For this review, take the finished solid that the model builds, in its own axes (mm). Round coordinates to 2 decimals unless told otherwise and drop trailing zeros. Write each loop counter-clockwise with the first axis right and the second up, starting at its lowest first coordinate (ties: lowest second). Pieces come first, ordered by that corner, then holes. Notation, with made-up numbers: M 61,84.25 L 104,84.25 A13 cw 104,103.25 Z; hole C 13,74.25 d2. An arc over 180 degrees is marked long. Use one line per item in the form item = value. Start each with the question number.
Item 1: For line 1 (X direction, y = 34.5, z = 1.8); line 2 (Y direction, x = 7, z = 2.25); line 3 (X direction, y = 5, z = 1.8), list the stretches that pass through material, from the lowest coordinate up. Write a range as [from, to].
Item 2: Draft analysis for pull direction Z (two halves, no side actions). For faces 1 (the flat face through (35, 22, 3)), 2 (the flat face through (69, 22, 2)), 3 (the flat face through (35, 22, 0)), state which applies: released by +Z, released by -Z, zero draft, split by the parting line, or undercut.
Item 3: For P1, Ø1.5, axis at x = 8.5, z = 2, coming from the +Y side, flat-tipped, find the tip position at first contact; note if it passes through.
Item 4: Add section A-A (z = 2.2). State the section outline as (x, y) points.
Autodesk Inventor part; units mm, degrees
ref_plane "YZ Plane" through (0, 0, 0) normal (1, 0, 0) x (0, 1, 0)
ref_plane "XZ Plane" through (0, 0, 0) normal (0, 1, 0) x (-1, 0, 0)
ref_plane "XY Plane" through (0, 0, 0) normal (0, 0, 1) x (1, 0, 0)
sketch "Boceto1" plane through (0, 0, 0) normal (0, 0, 1) x (1, 0, 0)
  line L0 (3, 0) -> (67, 0)
  line L1 (70, 3) -> (70, 41)
  line L2 (67, 44) -> (3, 44)
  line L3 (0, 41) -> (0, 3)
  arc A0 (3, 44) -> (0, 41) centre (3, 41) ccw
  arc A1 (0, 3) -> (3, 0) centre (3, 3) ccw
  arc A2 (67, 0) -> (70, 3) centre (67, 3) ccw
  arc A3 (70, 41) -> (67, 44) centre (67, 41) ccw
  point P0 (0, 0)
  point P1 (70, 44)
  point P2 (70, 0)
  point P3 (0, 44)
  dimension "d0" = 70
  dimension "d1" = 44
  dimension "d2" = 3
extrude "Extrusión1" add sketch "Boceto1" along normal blind 3
sketch "Boceto2" plane through (0, 0, 3) normal (0, 0, 1) x (1, 0, 0)
  line L0 (0, 41) -> (0, 3)
  arc A0 (0, 3) -> (3, 0) centre (3, 3) ccw
  line L1 (3, 0) -> (67, 0)
  arc A1 (67, 0) -> (70, 3) centre (67, 3) ccw
  line L2 (70, 3) -> (70, 41)
  arc A2 (70, 41) -> (67, 44) centre (67, 41) ccw
  line L3 (67, 44) -> (3, 44)
  arc A3 (3, 44) -> (0, 41) centre (3, 41) ccw
  line L4 (3, 43) -> (67, 43)
  arc A4 (69, 41) -> (67, 43) centre (67, 41) ccw
  line L5 (69, 41) -> (69, 3)
  arc A5 (67, 1) -> (69, 3) centre (67, 3) ccw
  line L6 (67, 1) -> (3, 1)
  arc A6 (1, 3) -> (3, 1) centre (3, 3) ccw
  line L7 (1, 3) -> (1, 41)
  arc A7 (3, 43) -> (1, 41) centre (3, 41) ccw
  point P0 (0, 0)
  dimension "d5" = 1
extrude "Extrusión2" cut sketch "Boceto2" against normal through all
sketch "Boceto5" plane through (0, 0, 3) normal (0, 0, 1) x (1, 0, 0)
  arc A0 (3, 43) -> (1, 41) centre (3, 41) ccw
  line L0 (1, 41) -> (1, 3)
  arc A1 (1, 3) -> (3, 1) centre (3, 3) ccw
  line L1 (3, 1) -> (67, 1)
  arc A2 (67, 1) -> (69, 3) centre (67, 3) ccw
  line L2 (69, 3) -> (69, 41)
  arc A3 (69, 41) -> (67, 43) centre (67, 41) ccw
  line L3 (67, 43) -> (3, 43)
  arc A4 (2.1716, 37.0858) -> (1, 34.2574) centre (5, 34.2574) ccw
  line L4 (1, 34.2574) -> (1, 9.7426)
  arc A5 (1, 9.7426) -> (2.1716, 6.9142) centre (5, 9.7426) ccw
  line L5 (2.1716, 6.9142) -> (6.9142, 2.1716)
  arc A6 (6.9142, 2.1716) -> (9.7426, 1) centre (9.7426, 5) ccw
  line L6 (9.7426, 1) -> (60.2574, 1)
  arc A7 (60.2574, 1) -> (63.0858, 2.1716) centre (60.2574, 5) ccw
  line L7 (63.0858, 2.1716) -> (67.8284, 6.9142)
  arc A8 (67.8284, 6.9142) -> (69, 9.7426) centre (65, 9.7426) ccw
  line L8 (69, 9.7426) -> (69, 34.2574)
  arc A9 (69, 34.2574) -> (67.8284, 37.0858) centre (65, 34.2574) ccw
  line L9 (67.8284, 37.0858) -> (63.0858, 41.8284)
  arc A10 (63.0858, 41.8284) -> (60.2574, 43) centre (60.2574, 39) ccw
  line L10 (60.2574, 43) -> (9.7426, 43)
  arc A11 (9.7426, 43) -> (6.9142, 41.8284) centre (9.7426, 39) ccw
  line L11 (6.9142, 41.8284) -> (2.1716, 37.0858)
  arc A12 (2.8787, 36.3787) -> (2, 34.2574) centre (5, 34.2574) ccw
  line L12 (2, 34.2574) -> (2, 9.7426)
  arc A13 (2, 9.7426) -> (2.8787, 7.6213) centre (5, 9.7426) ccw
  line L13 (2.8787, 7.6213) -> (7.6213, 2.8787)
  arc A14 (7.6213, 2.8787) -> (9.7426, 2) centre (9.7426, 5) ccw
  line L14 (9.7426, 2) -> (60.2574, 2)
  arc A15 (60.2574, 2) -> (62.3787, 2.8787) centre (60.2574, 5) ccw
  line L15 (62.3787, 2.8787) -> (67.1213, 7.6213)
  arc A16 (67.1213, 7.6213) -> (68, 9.7426) centre (65, 9.7426) ccw
  line L16 (68, 9.7426) -> (68, 34.2574)
  arc A17 (68, 34.2574) -> (67.1213, 36.3787) centre (65, 34.2574) ccw
  line L17 (67.1213, 36.3787) -> (62.3787, 41.1213)
  arc A18 (62.3787, 41.1213) -> (60.2574, 42) centre (60.2574, 39) ccw
  line L18 (60.2574, 42) -> (9.7426, 42)
  arc A19 (9.7426, 42) -> (7.6213, 41.1213) centre (9.7426, 39) ccw
  line L19 (7.6213, 41.1213) -> (2.8787, 36.3787)
  point P0 (0, 0)
  dimension "d0" = 70
  dimension "d1" = 44
  dimension "d2" = 3
  dimension "d23" = 1
  dimension "d24" = 4
  dimension "d25" = 8.7426
  dimension "d26" = 4
  dimension "d27" = 8.7426
  dimension "d28" = 4
  dimension "d29" = 4
  dimension "d30" = 8.7426
  dimension "d31" = 4
  dimension "d32" = 8.7426
  dimension "d33" = 4
  dimension "d34" = 4
  dimension "d35" = 8.7426
  dimension "d36" = 8.7426
  dimension "d37" = 4
  dimension "d38" = 8.7426
  dimension "d39" = 8.7426
  dimension "d40" = 4
  dimension "d41" = 4
  dimension "d42" = 4
  dimension "d43" = 1
  dimension "d44" = 1
  dimension "d45" = 4
  dimension "d46" = 4
  dimension "d47" = 1
  dimension "d48" = 4
  dimension "d49" = 4
  dimension "d50" = 4
  dimension "d51" = 45
  dimension "d52" = 45
  dimension "d53" = 45
  dimension "d54" = 45
  dimension "d55" = 90
  dimension "d56" = 90
extrude "Extrusión4" cut sketch "Boceto5" against normal through all contours L3 A11 L11 A4 L0 A0 | L3 A3 L2 A9 L9 A10 | A5 L5 A6 L1 A1 L0 | L2 A2 L1 A7 L7 A8
properties part number "3d_DAA - Enclosure Glass"
Calculated:
q1.line_1 = [1.01, 68.99]
q1.line_2 = [2.09, 41.91]
q1.line_3 = [4.09, 65.91]
q2.face_1 = released by +Z
q2.face_2 = zero draft
q2.face_3 = released by -Z
q3.P1 = 42.97
q4.outline = M 1,9.74 A4 ccw 2.17,6.91 L 6.91,2.17 A4 ccw 9.74,1 L 60.26,1 A4 ccw 63.09,2.17 L 67.83,6.91 A4 ccw 69,9.74 L 69,34.26 A4 ccw 67.83,37.09 L 63.09,41.83 A4 ccw 60.26,43 L 9.74,43 A4 ccw 6.91,41.83 L 2.17,37.09 A4 ccw 1,34.26 Z
